The drawing under review shows one solid part. Ordinate dimensions are in mm from its lowest x, y, z. A direction names the side the tool comes from. Coordinates: 2 decimals unless noted, no trailing zeros. Write each loop counter-clockwise with the first axis right and the second up, starting at its lowest first coordinate (ties: lowest second). Pieces come first, ordered by that corner, then holes.
1) For P1, Ø1.5, axis at x = 9, z = 7, coming from the +Y side; P2, Ø2, axis at x = 8.5, z = 9, coming from the -Y side, all flat-tipped, find the tip position at first contact; note any pin that passes through.
2) Machinability: for the marked faces 3, 4 and 5, which of the approach directions +Z, -Z, +X, -X, +Y, -Y give a long, thin tool a straight path to every point of the face, cutting with its end or side? Answer none if there is none.
3) Add section A-A, the plane y = 12.25. State the section outline as (x, z) points, then the cut area to 3 significant figures.
4) Add section C-C, the plane z = 2. State the section outline as (x, y) points.
5) For line 1 (X direction, y = 17, z = 6.25), list the stretches that pass through material, from the lowest coordinate up.
6) Add section D-D, the plane x = 4.5. State the section outline as (y, z) points, then the cut area to 3 significant figures.
7) Add section B-B, the plane x = 10. State the section outline as (y, z) points.
8) Mouldability with a two-part tool opening along Y and no side actions: class the marked faces 1 and 2 as released by +Y, released by -Y, zero draft, split by the parting line, or undercut.
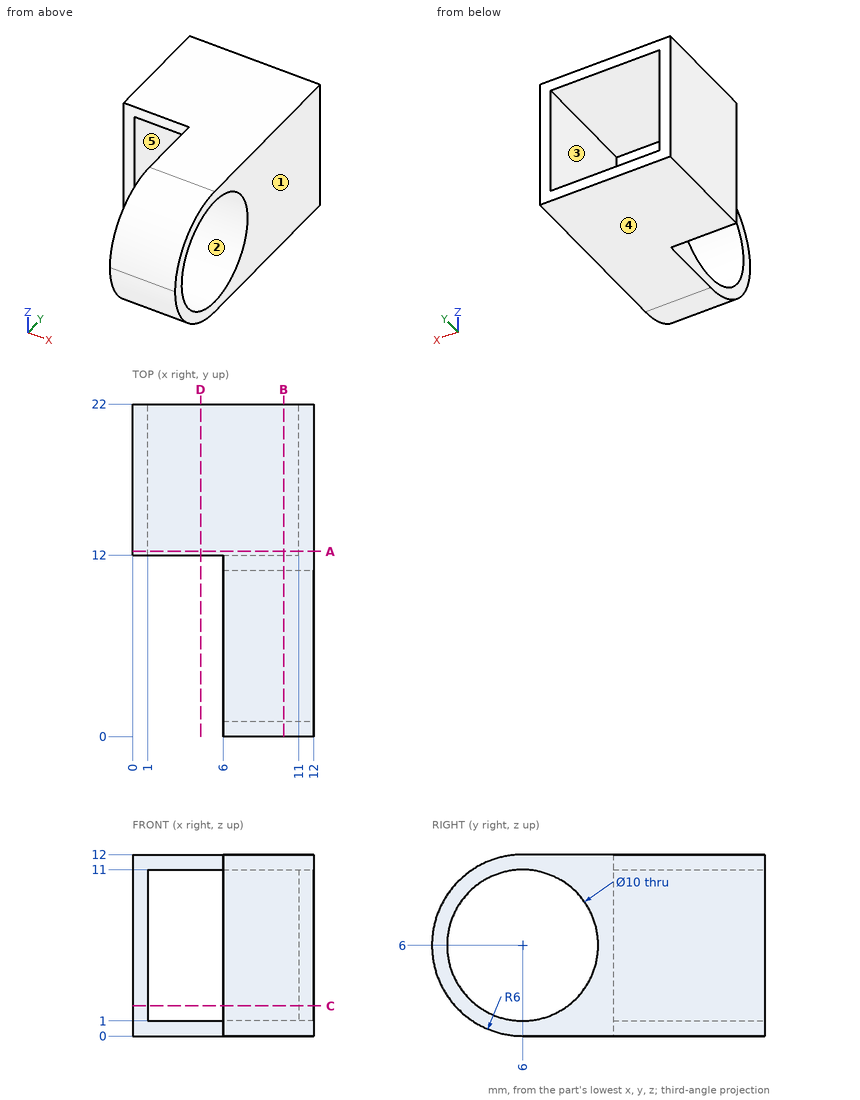
Geometry results:
1. P1: stops at y = 12
1. P2: stops at y = 0.34
2. face 3: +Y
2. face 4: -Z, +X, -X, +Y, -Y
2. face 5: +Y, -Y
3. outline: (0, 0) - (12, 0) - (12, 12) - (0, 12) - close; hole (1, 1) - (11, 1) - (11, 11) - (1, 11) - close
3. area: 44.0 mm2
4. outline: (0, 12) - (1, 12) - (1, 22) - (0, 22) - close; (6, 1.53) - (12, 1.53) - (12, 3) - (6, 3) - close; (6, 9) - (12, 9) - (12, 22) - (11, 22) - (11, 12) - (6, 12) - close
5. line 1: x = 0 to 1, 11 to 12
6. outline: (12, 0) - (22, 0) - (22, 1) - (12, 1) - close; (12, 11) - (22, 11) - (22, 12) - (12, 12) - close
6. area: 20.0 mm2
7. outline: (6, 0) - (22, 0) - (22, 1) - (12, 1) - (12, 11) - (22, 11) - (22, 12) - (6, 12) arc R6 ccw to start; hole circle Ø10 at (6, 6)
8. face 1: zero draft
8. face 2: undercut
